Verification items for the finished model (mm, model axes). A direction names the side the tool comes from. Give positions to 0.01 mm unless a question says otherwise; leave off trailing zeros. Loops run counter-clockwise (first coordinate to the right, second up) from the corner with the lowest first, then second, coordinate; pieces in that order, holes last. Notation, with made-up numbers: (-7.5, -1) - (7.5, -1) arc R19 ccw to (7.5, 10) - close; hole circle Ø3 at (75.25, -4). An arc over 180 degrees is marked (long way). One line per item, written item: value. Start each with the question number.
1. Gauge pin test, flat ends, axial feed: pin 1 (1 mm diameter, centred on x = -37.5, z = 2, fed in from +Y); pin 2 (2.5 mm diameter, centred on y = 30, z = 2, fed in from -X). Record the tip position at first contact, or that the pin passes through.
2. Mould release check, pull along Y, two halves, no side actions. Record for faces 1 (the flat face through (-1, -15, 0)), 2 (the flat face through (74.33, -114.29, 2.46)), 3 (the flat face through (1, -41.068, 2)): pulls with the +Y half, pulls with the -Y half, needs draft (parallel to the pull), parting line crosses it, or undercut.
3. Scan lines: L1, parallel to Y at x = -0.5, z = 2.55; L2, parallel to X at y = -56, z = 4.25; L3, parallel to Y at x = -7, z = 1.4. Record each from-to range of solid material in increasing order. Write a range as [from, to].
4. Access from +Z, -Z, +X, -X, +Y, -Y to the whole of each face (thin tool, end or side, straight path). Record for faces 4 (the flat face through (74, -99.185, 2)), 5 (the flat face through (-75, -99.743, 2)), 6 (the flat face through (46, -108.2, 2)), 7 (the flat face through (-66.5, -104.01, 2.46)), 8 (the cylindrical face through (-63.69, 78.34, 2.46)).
5. Sectioned sample at B-B (y = -11). Count the separate pieces of the cut face and the enclosed holes in it, plus the area to 3 significant figures.
6. Sectioned sample at A-A (x = 18.5). Record the cut outline in (y, z), plus the area to 3 significant figures.
from build123d import *

# Parameters (mm, degrees)
SKETCH1_W           = 20
SKETCH1_H           = 4
SKETCH1_W_2         = 17.635389858
SKETCH1_H_2         = 3.879785769
SKETCH1_W_3         = 4.102446126
SKETCH1_H_3         = 20.774322756
SKETCH1_H_4         = 21.660832558
SKETCH1_W_4         = 3.418162198
SKETCH1_H_5         = 5.631856247
SKETCH1_W_5         = 16.224558669
BOSS_EXTRUDE3_DEPTH = 5


with BuildPart() as part:
    # Sketch1 → Boss-Extrude3 (new body)
    with BuildSketch(Plane.XY):
        with BuildLine():
            Line((-46.908869484, -52.720617246), (-28.908869484, -52.720617246))
            ThreePointArc((-28.908869484, -52.720617246), (-27.586230621, -53.216332062), (-26.915218553, -54.459251828))
            add(Edge.make_bspline(
                [(-27.150183285, -104.622936523), (-24.042180825, -75.385235173), (-26.915218553, -54.459251828)],
                knots=[4.03312472, 4.03312472, 4.03312472, 5.695988701, 5.695988701, 5.695988701], degree=2, weights=[1, 0.673818357, 1]))
            ThreePointArc((-27.150183285, -104.622936523), (-28.453010553, -107.174276905), (-31.127773146, -108.200113985))
            Line((-31.127773146, -108.200113985), (-61.691034949, -108.200113985))
            ThreePointArc((-61.691034949, -108.200113985), (-62.986836684, -107.905829762), (-64.028415748, -107.080712561))
            Line((-64.028415748, -107.080712561), (-69.031690033, -100.862183312))
            ThreePointArc((-69.031690033, -100.862183312), (-70.073269096, -100.037066111), (-71.369070832, -99.742781887))
            Line((-71.369070832, -99.742781887), (-77.798044438, -99.742781887))
            ThreePointArc((-77.798044438, -99.742781887), (-80.408451089, -101.264344498), (-80.370926301, -104.285597145))
            Line((-80.370926301, -104.285597145), (-68.103793269, -124.742929243))
            ThreePointArc((-68.103793269, -124.742929243), (-67.009348795, -125.810520637), (-65.530911406, -126.200113985))
            Line((-65.530911406, -126.200113985), (65.997283419, -126.200113985))
            ThreePointArc((65.997283419, -126.200113985), (67.523464533, -125.782897602), (68.625147136, -124.647294791))
            Line((68.625147136, -124.647294791), (80.198497538, -103.631822855))
            ThreePointArc((80.198497538, -103.631822855), (80.153417437, -100.658460936), (77.570633821, -99.18464205))
            Line((77.570633821, -99.18464205), (69.904360471, -99.18464205))
            ThreePointArc((69.904360471, -99.18464205), (68.383344987, -99.598812996), (67.282303117, -100.726967452))
            Line((67.282303117, -100.726967452), (63.985194726, -106.657788583))
            ThreePointArc((63.985194726, -106.657788583), (62.884152857, -107.785943039), (61.363137372, -108.200113985))
            Line((61.363137372, -108.200113985), (31.127773146, -108.200113985))
            ThreePointArc((31.127773146, -108.200113985), (28.453010553, -107.174276905), (27.150183285, -104.622936523))
            add(Edge.make_bspline(
                [(26.915218553, -54.459251828), (24.042180825, -75.385235173), (27.150183285, -104.622936523)],
                knots=[0.587196606, 0.587196606, 0.587196606, 2.250060588, 2.250060588, 2.250060588], degree=2, weights=[1, 0.673818357, 1]))
            ThreePointArc((26.915218553, -54.459251828), (27.586230621, -53.216332062), (28.908869484, -52.720617246))
            Line((28.908869484, -52.720617246), (46.908869484, -52.720617246))
            ThreePointArc((46.908869484, -52.720617246), (49.976562122, -51.287573006), (50.846185128, -48.015248183))
            add(Edge.make_bspline(
                [(49.632919584, 69.157622076), (40.820331779, 7.94829107), (50.846185128, -48.015248183)],
                knots=[0.92694213, 0.92694213, 0.92694213, 2.321414523, 2.321414523, 2.321414523], degree=2, weights=[1, 0.766619755, 1]))
            ThreePointArc((49.632919584, 69.157622076), (49.855189189, 69.656136563), (50.306120041, 69.963678167))
            ThreePointArc((50.306120041, 69.963678167), (55.512793259, 71.035230988), (60.82526432, 70.847287719))
            ThreePointArc((60.82526432, 70.847287719), (61.349200112, 70.906348269), (61.770271319, 71.223674443))
            ThreePointArc((61.770271319, 71.223674443), (63.704662293, 78.231916543), (60.165141812, 84.582437823))
            ThreePointArc((60.165141812, 84.582437823), (0, 93.879837075), (-60.165141812, 84.582437823))
            ThreePointArc((-60.165141812, 84.582437823), (-63.704662293, 78.231916543), (-61.770271319, 71.223674443))
            ThreePointArc((-61.770271319, 71.223674443), (-61.349200112, 70.906348269), (-60.82526432, 70.847287719))
            ThreePointArc((-60.82526432, 70.847287719), (-55.512793259, 71.035230988), (-50.306120041, 69.963678167))
            ThreePointArc((-50.306120041, 69.963678167), (-49.855189189, 69.656136563), (-49.632919584, 69.157622076))
            add(Edge.make_bspline(
                [(-50.846185128, -48.015248183), (-40.820331779, 7.94829107), (-49.632919584, 69.157622076)],
                knots=[3.961770785, 3.961770785, 3.961770785, 5.356243177, 5.356243177, 5.356243177], degree=2, weights=[1, 0.766619755, 1]))
            ThreePointArc((-50.846185128, -48.015248183), (-49.976562122, -51.287573006), (-46.908869484, -52.720617246))
        make_face()
        with Locations((1.663675391, 80.068012143)):
            Rectangle(SKETCH1_W, SKETCH1_H, mode=Mode.SUBTRACT)
        with Locations((13.088476945, -57.636754326)):
            Rectangle(SKETCH1_W_2, SKETCH1_H_2, mode=Mode.SUBTRACT)
        with Locations((38.10837085, 31.531905503)):
            Rectangle(SKETCH1_W_3, SKETCH1_H_3, mode=Mode.SUBTRACT)
        with Locations((38.10837085, -2.949787997)):
            Rectangle(SKETCH1_W_3, SKETCH1_H_4, mode=Mode.SUBTRACT)
        with Locations((-37.615690315, 30.327596937)):
            Rectangle(SKETCH1_W_4, SKETCH1_H_3, mode=Mode.SUBTRACT)
        with Locations((-36.862997462, -3.250865139)):
            Rectangle(SKETCH1_W_4, SKETCH1_H_4, mode=Mode.SUBTRACT)
        with Locations((1.610001599, -43.883655008)):
            Rectangle(SKETCH1_W, SKETCH1_H_5, mode=Mode.SUBTRACT)
        with Locations((-13.978236501, -57.624038848)):
            Rectangle(SKETCH1_W_5, SKETCH1_H_2, mode=Mode.SUBTRACT)
    extrude(amount=BOSS_EXTRUDE3_DEPTH)


solid = part.part
Results are:
1. pin 1: stops at y = 90.42
1. pin 2: stops at x = -46.43
2. face 1: needs draft
2. face 2: pulls with the -Y half
2. face 3: undercut
3. L1: y = [-126.2, -46.7], [-41.07, 78.07], [82.07, 93.88]
3. L2: x = [-26.72, -22.09], [-5.87, 4.27], [21.91, 26.72]
3. L3: y = [-126.2, -59.56], [-55.68, -46.7], [-41.07, 78.07], [82.07, 93.76]
4. face 4: +Z, -Z, +X, +Y
4. face 5: +Z, -Z, -X, +Y
4. face 6: +Z, -Z
4. face 7: +Z, -Z, +Y
4. face 8: +Z, -Z, -X
5. separate pieces: 3
5. enclosed holes: 0
5. area: 431 mm^2
6. outline: (-126.2, 0) - (-59.58, 0) - (-59.58, 5) - (-126.2, 5) - close; (-55.7, 0) - (93.02, 0) - (93.02, 5) - (-55.7, 5) - close
6. area: 1,080 mm^2
